Here's how the part is built. I have some questions about the finished solid (model axes, mm). A direction names the side the tool comes from. Coordinates: 2 decimals unless noted, no trailing zeros. Loops run counter-clockwise (first coordinate to the right, second up) from the corner with the lowest first, then second, coordinate; pieces in that order, holes last. Notation, with made-up numbers: (37, -20) -> (59, -20) arc R16 ccw to (59, 3) -> close; hole circle Ø4 at (-24, 30.25). An arc over 180 degrees is marked (long way). Use CSV: the item, a comma, the result in double quotes. Start each with the question number.
from build123d import *

# Parameters (mm, degrees)
BOSS_EXTRUDE1_DEPTH = 38.1
SKETCH4_W           = 8.89
SKETCH4_H           = 6.35
CUT_EXTRUDE1_DEPTH  = 8.89
SKETCH5_W           = 6.35
SKETCH5_H           = 8.89
CUT_EXTRUDE2_DEPTH  = 40.132
SKETCH6_R           = 2.2479
CUT_EXTRUDE3_DEPTH  = 74.93
CUT_EXTRUDE8_START  = -11.43
SKETCH10_R          = 3.937
CUT_EXTRUDE8_DEPTH  = 11.43


with BuildPart() as part:
    # Sketch1 → Boss-Extrude1 (new body)
    with BuildSketch(Plane.XY):
        with BuildLine():
            Line((0, 0), (50.8, 0))
            Line((50.8, 0), (50.8, 35.56))
            ThreePointArc((50.8, 35.56), (50.056051224, 37.356051224), (48.26, 38.1))
            Line((48.26, 38.1), (32.010551811, 38.1))
            ThreePointArc((32.010551811, 38.1), (31.24675908, 37.982441055), (30.553667663, 37.640646192))
            Line((30.553667663, 37.640646192), (1.083115852, 17.005143659))
            ThreePointArc((1.083115852, 17.005143659), (0.286992484, 16.097338944), (0, 14.924497467))
            Line((0, 14.924497467), (0, 0))
        make_face()
    extrude(amount=BOSS_EXTRUDE1_DEPTH)

    # Sketch4 → Cut-Extrude1 (cut)
    with BuildSketch(Plane(origin=(-7.6334698, 10.901724679, 0), x_dir=(0.819152044, 0.573576436, 0), z_dir=(-0.573576436, 0.819152044, 0))):
        with Locations((20.625340071, -32.385)):
            Rectangle(SKETCH4_W, SKETCH4_H)
    extrude(amount=-CUT_EXTRUDE1_DEPTH, mode=Mode.SUBTRACT)

    # Sketch5 → Cut-Extrude2 (cut)
    with BuildSketch(Plane(origin=(50.8, 0, 0), x_dir=(0, 0, -1), z_dir=(1, 0, 0))):
        with Locations((-32.385, 17.345124802)):
            Rectangle(SKETCH5_W, SKETCH5_H)
    extrude(amount=-CUT_EXTRUDE2_DEPTH, mode=Mode.SUBTRACT)

    # Sketch6 → Cut-Extrude3 (cut)
    with BuildSketch(Plane.XZ):
        with Locations((44.214054574, 23.424710834)):
            Circle(SKETCH6_R)
        with Locations((10.414, 10.922)):
            Circle(SKETCH6_R)
    extrude(amount=-CUT_EXTRUDE3_DEPTH, mode=Mode.SUBTRACT)

    # Sketch10 → Cut-Extrude8 (cut)
    with BuildSketch(Plane(origin=(0, 38.1, 0), x_dir=(1, 0, 0), z_dir=(0, 1, 0)).offset(CUT_EXTRUDE8_START)):
        with Locations((10.414, -10.922)):
            Circle(SKETCH10_R)
    extrude(amount=-CUT_EXTRUDE8_DEPTH, mode=Mode.SUBTRACT)


solid = part.part
1) Please list where these lines run through material, in increasing order: L1, parallel to Z at x = 45.5, y = 21.5; L2, parallel to Y at x = 10.5, z = 8; L3, parallel to Y at x = 36, z = 32. Write a range as [from, to].
2) I want a section at A-A, the plane z = 30.5. Please give me the cut outline in (x, y).
3) I want a section at B-B, the plane x = 41. Please give me the cut outline in (y, z).
4) Thinking about a two-plate mould opening in Y: for faces 6 (the face through (14.17, 19.62, 9.74)), 7 (the face through (16.025, 27.467, 18.783)), 8 (the face through (33, 21.79, 32)), which applies, pulls with the +Y half, pulls with the -Y half, needs draft (parallel to the pull), parting line crosses it, or undercut?
5) I want a section at C-C, the plane y = 3.5. Please give me the cut outline in (x, z).
6) I want a section at D-D, the plane z = 5. Please give me the cut outline in (x, y), plus the area to 3 significant figures.
7) For P1, Ø8, axis at x = 28, z = 30.5, coming from the +Y side; P2, Ø6.5, axis at x = 12, z = 11, coming from the +Y side; P3, Ø4, axis at x = 11.5, z = 5, coming from the +Y side; P4, Ø1.9, axis at x = 28, z = 32, coming from the +Y side, each with a flat end and sliding along its axis, tell me the tip position at first contact or that it passes through.
8) Which directions (+Z, -Z, +X, -X, +Y, -Y) give clear straight access to the entire face, cutting with the end or side of a thin tool? Please do faces 1 (the face through (12.49, 7.51, 10.06)), 2 (the face through (8.11, 16.63, 32.43)), 3 (the face through (12, 15.24, 13)), 4 (the face through (31, 12.9, 32)), 5 (the face through (14.11, 23.56, 32.43)).
Return value:
1,L1,"z = [0, 21.58], [25.27, 29.21], [35.56, 38.1]"
1,L2,"y = [0, 15.24]"
1,L3,"y = [0, 12.9], [21.79, 38.1]"
2,outline,"(0, 0) -> (50.8, 0) -> (50.8, 12.9) -> (10.67, 12.9) -> (10.67, 12.97) -> (5.62, 20.18) -> (1.08, 17.01) arc R2.54 ccw to (0, 14.92) -> close; (12.9, 25.28) -> (15.35, 21.79) -> (50.8, 21.79) -> (50.8, 35.56) arc R2.54 ccw to (48.26, 38.1) -> (32.01, 38.1) arc R2.54 ccw to (30.55, 37.64) -> close"
3,outline,"(0, 0) -> (38.1, 0) -> (38.1, 38.1) -> (0, 38.1) -> close; hole (12.9, 29.21) -> (21.79, 29.21) -> (21.79, 35.56) -> (12.9, 35.56) -> close"
4,face 6,"needs draft"
4,face 7,"pulls with the +Y half"
4,face 8,"undercut"
5,outline,"(0, 0) -> (50.8, 0) -> (50.8, 38.1) -> (0, 38.1) -> close; hole circle Ø4.5 at (10.41, 10.92); hole circle Ø4.5 at (44.21, 23.42)"
6,outline,"(0, 0) -> (50.8, 0) -> (50.8, 35.56) arc R2.54 ccw to (48.26, 38.1) -> (32.01, 38.1) arc R2.54 ccw to (30.55, 37.64) -> (1.08, 17.01) arc R2.54 ccw to (0, 14.92) -> close"
6,area,"1,590 mm²"
7,P1,"stops at y = 38.1"
7,P2,"stops at y = 26.92"
7,P3,"stops at y = 25.7"
7,P4,"stops at y = 36.52"
8,face 1,"+Y, -Y"
8,face 2,"+X, +Y"
8,face 3,"+Y"
8,face 4,"+X"
8,face 5,"-X"
